Input: part model. Units: mm. Frame: model coordinates. Round coordinates to 2 decimals unless told otherwise and drop trailing zeros. Order: outer loops, then holes, each group sorted by start corner. A loop starts at its lowest first (then second) coordinate and runs counter-clockwise, first axis right, second up. Notation, with made-up numbers: (45, -30.75) -> (89, -30.75) arc R25 ccw to (89, -5.75) -> close; hole circle Ø11 at (68.25, 24). An arc over 180 degrees is marked (long way). Use a Markdown table: item, result.
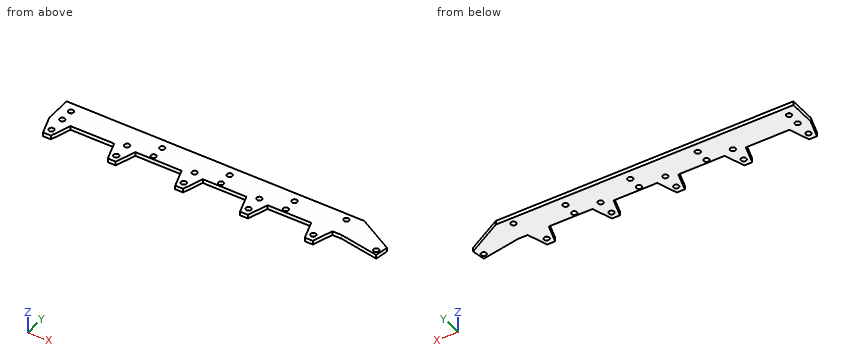
from build123d import *

# Parameters (mm, degrees)
CYLINDER012_R     = 2
CYLINDER012_DEPTH = 10
CYLINDER013_R     = 2
CYLINDER013_DEPTH = 10
CYLINDER014_R     = 2
CYLINDER014_DEPTH = 10
CYLINDER015_R     = 2
CYLINDER015_DEPTH = 10
CYLINDER016_R     = 2
CYLINDER016_DEPTH = 10
CYLINDER017_R     = 2
CYLINDER017_DEPTH = 10
CYLINDER018_R     = 2
CYLINDER018_DEPTH = 10
CYLINDER011_R     = 2
CYLINDER011_DEPTH = 10
CYLINDER007_R     = 2
CYLINDER007_DEPTH = 10
CYLINDER008_R     = 2
CYLINDER008_DEPTH = 10
CYLINDER009_R     = 2
CYLINDER009_DEPTH = 10
CYLINDER010_R     = 2
CYLINDER010_DEPTH = 10
CYLINDER006_R     = 2
CYLINDER006_DEPTH = 10
CYLINDER001_R     = 2
CYLINDER001_DEPTH = 10
CYLINDER005_R     = 2
CYLINDER005_DEPTH = 10
CYLINDER004_R     = 2
CYLINDER004_DEPTH = 10
CYLINDER003_R     = 2
CYLINDER003_DEPTH = 10
CYLINDER002_R     = 2
CYLINDER002_DEPTH = 10
CYLINDER_R        = 2
CYLINDER_DEPTH    = 10
PAD_DEPTH         = 3


with BuildPart() as cylinder012:
    # Cylinder012 → Cylinder012 (new body)
    with BuildSketch(Plane(origin=(37.5, -6.5, -5), x_dir=(1, 0, 0), z_dir=(0, 0, 1))):
        Circle(CYLINDER012_R)
    extrude(amount=CYLINDER012_DEPTH)


with BuildPart() as cylinder013:
    # Cylinder013 → Cylinder013 (new body)
    with BuildSketch(Plane(origin=(88.5, 3.5, -5), x_dir=(1, 0, 0), z_dir=(0, 0, 1))):
        Circle(CYLINDER013_R)
    extrude(amount=CYLINDER013_DEPTH)


with BuildPart() as cylinder014:
    # Cylinder014 → Cylinder014 (new body)
    with BuildSketch(Plane(origin=(88.5, -6.5, -5), x_dir=(1, 0, 0), z_dir=(0, 0, 1))):
        Circle(CYLINDER014_R)
    extrude(amount=CYLINDER014_DEPTH)


with BuildPart() as cylinder015:
    # Cylinder015 → Cylinder015 (new body)
    with BuildSketch(Plane(origin=(137.5, -6.5, -5), x_dir=(1, 0, 0), z_dir=(0, 0, 1))):
        Circle(CYLINDER015_R)
    extrude(amount=CYLINDER015_DEPTH)


with BuildPart() as cylinder016:
    # Cylinder016 → Cylinder016 (new body)
    with BuildSketch(Plane(origin=(137.5, 3.5, -5), x_dir=(1, 0, 0), z_dir=(0, 0, 1))):
        Circle(CYLINDER016_R)
    extrude(amount=CYLINDER016_DEPTH)


with BuildPart() as cylinder017:
    # Cylinder017 → Cylinder017 (new body)
    with BuildSketch(Plane(origin=(37.5, 3.5, -5), x_dir=(1, 0, 0), z_dir=(0, 0, 1))):
        Circle(CYLINDER017_R)
    extrude(amount=CYLINDER017_DEPTH)


with BuildPart() as cylinder018:
    # Cylinder018 → Cylinder018 (new body)
    with BuildSketch(Plane(origin=(117.5, -6.5, -5), x_dir=(1, 0, 0), z_dir=(0, 0, 1))):
        Circle(CYLINDER018_R)
    extrude(amount=CYLINDER018_DEPTH)


with BuildPart() as cylinder011:
    # Cylinder011 → Cylinder011 (new body)
    with BuildSketch(Plane(origin=(-31.5, 3.5, -5), x_dir=(1, 0, 0), z_dir=(0, 0, 1))):
        Circle(CYLINDER011_R)
    extrude(amount=CYLINDER011_DEPTH)


with BuildPart() as cylinder007:
    # Cylinder007 → Cylinder007 (new body)
    with BuildSketch(Plane(origin=(117.5, -6.5, -3), x_dir=(1, 0, 0), z_dir=(0, 0, 1))):
        Circle(CYLINDER007_R)
    extrude(amount=CYLINDER007_DEPTH)


with BuildPart() as cylinder008:
    # Cylinder008 → Cylinder008 (new body)
    with BuildSketch(Plane(origin=(68.5, -6.5, -3), x_dir=(1, 0, 0), z_dir=(0, 0, 1))):
        Circle(CYLINDER008_R)
    extrude(amount=CYLINDER008_DEPTH)


with BuildPart() as cylinder009:
    # Cylinder009 → Cylinder009 (new body)
    with BuildSketch(Plane(origin=(17.5, -6.5, -3), x_dir=(1, 0, 0), z_dir=(0, 0, 1))):
        Circle(CYLINDER009_R)
    extrude(amount=CYLINDER009_DEPTH)


with BuildPart() as cylinder010:
    # Cylinder010 → Cylinder010 (new body)
    with BuildSketch(Plane(origin=(-31.5, -6.5, -3), x_dir=(1, 0, 0), z_dir=(0, 0, 1))):
        Circle(CYLINDER010_R)
    extrude(amount=CYLINDER010_DEPTH)


with BuildPart() as cylinder006:
    # Cylinder006 → Cylinder006 (new body)
    with BuildSketch(Plane(origin=(175.5, 5.5, -3), x_dir=(1, 0, 0), z_dir=(0, 0, 1))):
        Circle(CYLINDER006_R)
    extrude(amount=CYLINDER006_DEPTH)


with BuildPart() as cylinder001:
    # Cylinder001 → Cylinder001 (new body)
    with BuildSketch(Plane(origin=(166.5, -19, -3), x_dir=(1, 0, 0), z_dir=(0, 0, 1))):
        Circle(CYLINDER001_R)
    extrude(amount=CYLINDER001_DEPTH)


with BuildPart() as cylinder005:
    # Cylinder005 → Cylinder005 (new body)
    with BuildSketch(Plane(origin=(208.5, -10.5, -3), x_dir=(1, 0, 0), z_dir=(0, 0, 1))):
        Circle(CYLINDER005_R)
    extrude(amount=CYLINDER005_DEPTH)


with BuildPart() as cylinder004:
    # Cylinder004 → Cylinder004 (new body)
    with BuildSketch(Plane(origin=(-31.5, -19, -3), x_dir=(1, 0, 0), z_dir=(0, 0, 1))):
        Circle(CYLINDER004_R)
    extrude(amount=CYLINDER004_DEPTH)


with BuildPart() as cylinder003:
    # Cylinder003 → Cylinder003 (new body)
    with BuildSketch(Plane(origin=(68.5, -19, -3), x_dir=(1, 0, 0), z_dir=(0, 0, 1))):
        Circle(CYLINDER003_R)
    extrude(amount=CYLINDER003_DEPTH)


with BuildPart() as cylinder002:
    # Cylinder002 → Cylinder002 (new body)
    with BuildSketch(Plane(origin=(117.5, -19, -3), x_dir=(1, 0, 0), z_dir=(0, 0, 1))):
        Circle(CYLINDER002_R)
    extrude(amount=CYLINDER002_DEPTH)


with BuildPart() as cylinder:
    # Cylinder → Cylinder (new body)
    with BuildSketch(Plane(origin=(17.5, -19, -3), x_dir=(1, 0, 0), z_dir=(0, 0, 1))):
        Circle(CYLINDER_R)
    extrude(amount=CYLINDER_DEPTH)


with BuildPart() as cut018:
    # Sketch001 → Pad (new body)
    with BuildSketch(Plane.XY):
        Polygon((-43.448801, 7.664407), (181.551199, 7.664407), (208.831914, -7.696961), (207.095432, -17.545038), (177.551199, -12.335593), (170.551199, -12.335593), (165.551199, -27.335593), (159.551199, -27.335593), (154.551199, -12.335593), (121.551199, -12.335593), (116.551199, -27.335593), (110.551199, -27.335593), (105.551199, -12.335593), (72.551199, -12.335593), (67.551199, -27.335593), (61.551199, -27.335593), (56.551199, -12.335593), (21.551199, -12.335593), (16.551199, -27.335593), (10.551199, -27.335593), (5.551199, -12.335593), (-27.448801, -12.335593), (-32.448801, -27.335593), (-38.448801, -27.335593), (-43.448801, -12.335593), align=None)
    extrude(amount=PAD_DEPTH)


with BuildPart() as cut018_1:
    # Body001 placement: moved
    add(cut018.part.moved(Location((4, 3, 0))))

    # Cut: cut Cylinder
    add(cylinder.part, mode=Mode.SUBTRACT)

    # Cut001: cut Cylinder002
    add(cylinder002.part, mode=Mode.SUBTRACT)

    # Cut002: cut Cylinder003
    add(cylinder003.part, mode=Mode.SUBTRACT)

    # Cut003: cut Cylinder004
    add(cylinder004.part, mode=Mode.SUBTRACT)

    # Cut004: cut Cylinder005
    add(cylinder005.part, mode=Mode.SUBTRACT)

    # Cut005: cut Cylinder001
    add(cylinder001.part, mode=Mode.SUBTRACT)

    # Cut006: cut Cylinder006
    add(cylinder006.part, mode=Mode.SUBTRACT)

    # Cut007: cut Cylinder010
    add(cylinder010.part, mode=Mode.SUBTRACT)

    # Cut008: cut Cylinder009
    add(cylinder009.part, mode=Mode.SUBTRACT)

    # Cut009: cut Cylinder008
    add(cylinder008.part, mode=Mode.SUBTRACT)

    # Cut010: cut Cylinder007
    add(cylinder007.part, mode=Mode.SUBTRACT)

    # Cut011: cut Cylinder011
    add(cylinder011.part, mode=Mode.SUBTRACT)

    # Cut012: cut Cylinder018
    add(cylinder018.part, mode=Mode.SUBTRACT)

    # Cut013: cut Cylinder017
    add(cylinder017.part, mode=Mode.SUBTRACT)

    # Cut014: cut Cylinder016
    add(cylinder016.part, mode=Mode.SUBTRACT)

    # Cut015: cut Cylinder015
    add(cylinder015.part, mode=Mode.SUBTRACT)

    # Cut016: cut Cylinder014
    add(cylinder014.part, mode=Mode.SUBTRACT)

    # Cut017: cut Cylinder013
    add(cylinder013.part, mode=Mode.SUBTRACT)

    # Cut018: cut Cylinder012
    add(cylinder012.part, mode=Mode.SUBTRACT)


solid = cut018_1.part
1) Cut plane A-A on x = 33. Return loops of the section in (y, z).
Answer key:
| item | result |
|---|---|
| outline | (-9.34, 0) -> (10.66, 0) -> (10.66, 3) -> (-9.34, 3) -> close |
2) Contact query for a flat-ended pin moving along its axis: P1, Ø1.5, axis at x = 179, z = 1.5, coming from the -Y side. Output: stop coordinate, or through.
Answer key:
| item | result |
|---|---|
| P1 | stops at y = -9.34 |
3) Ray query, probe 1 along Y at (x, z) = (-31.5, 1.75); probe 2 along Y at (x, z) = (37.5, 1.2); probe 3 along Y at (x, z) = (175.5, 1.25). Return the intervals inside material, ascending.
Answer key:
| item | result |
|---|---|
| probe 1 | y = -24.34 to -21, -17 to -8.5, -4.5 to 1.5, 5.5 to 10.66 |
| probe 2 | y = -9.34 to -8.5, -4.5 to 1.5, 5.5 to 10.66 |
| probe 3 | y = -9.34 to 3.5, 7.5 to 10.66 |
4) Cut plane B-B on z = 1.1. State how many separate pieces and enclosed holes the cut face has, and give its area (3 significant figures).
Answer key:
| item | result |
|---|---|
| separate pieces | 1 |
| enclosed holes | 18 |
| area | 5,510 mm^2 |
5) Cut plane C-C on x = 63. Return loops of the section in (y, z), and give its area (3 significant figures).
Answer key:
| item | result |
|---|---|
| outline | (-16.68, 0) -> (10.66, 0) -> (10.66, 3) -> (-16.68, 3) -> close |
| area | 82.0 mm^2 |
